Model file for the job. Use its own axes, mm. A direction names the side the tool comes from. Round coordinates to 2 decimals unless told otherwise and drop trailing zeros. Write each loop counter-clockwise with the first axis right and the second up, starting at its lowest first coordinate (ties: lowest second). Pieces come first, ordered by that corner, then holes. Notation, with made-up numbers: (36, 11.5) - (59, 11.5) arc R24 ccw to (59, 36.5) - close; hole circle Ø2 at (52, -9.75). An arc over 180 degrees is marked (long way). One line per item, written item: value.
from build123d import *

# Parameters (mm, degrees)
SKETCH_1_W          = 54
SKETCH_1_H          = 48
EXTRUDE_1_DEPTH     = 1
SKETCH_2_R          = 1.5
CUT_EXTRUDE_1_DEPTH = 37.138621999
FILLET_1_R          = 5
SKETCH_3_W          = 10
SKETCH_3_H          = 7
EXTRUDE_2_DEPTH     = 5
SKETCH_4_W          = 8
SKETCH_4_H          = 8
SKETCH_4_W_2        = 4
SKETCH_4_H_2        = 6
SKETCH_4_H_3        = 4
EXTRUDE_3_DEPTH     = 1


with BuildPart() as part:
    # ｽｹｯﾁ1 → ﾎﾞｽ - 押し出し1 (new body)
    with BuildSketch(Plane.XY):
        Rectangle(SKETCH_1_W, SKETCH_1_H)
    extrude(amount=EXTRUDE_1_DEPTH)

    # ｽｹｯﾁ2 → ｶｯﾄ - 押し出し1 (cut, through all)
    with BuildSketch(Plane.XY.offset(1)):
        with Locations((-24.5, 21)):
            Circle(SKETCH_2_R)
        with Locations((24.5, -21)):
            Circle(SKETCH_2_R)
    extrude(amount=-CUT_EXTRUDE_1_DEPTH, mode=Mode.SUBTRACT)

    # ﾌｨﾚｯﾄ1
    fillet_1_edges = [part.edges().sort_by_distance(p)[0] for p in [
        (27, -24, 0.5),
        (-27, -24, 0.5),
        (-27, 24, 0.5),
        (27, 24, 0.5),
    ]]
    fillet(fillet_1_edges, radius=FILLET_1_R)

    # ｽｹｯﾁ3 → ﾎﾞｽ - 押し出し2 (add)
    with BuildSketch(Plane.XY.offset(1)):
        with Locations((-14, 19.5)):
            Rectangle(SKETCH_3_W, SKETCH_3_H)
        with Locations((0, 19.5)):
            Rectangle(SKETCH_3_W, SKETCH_3_H)
        with Locations((14, 19.5)):
            Rectangle(SKETCH_3_W, SKETCH_3_H)
        with Locations((-14, -19.5)):
            Rectangle(SKETCH_3_W, SKETCH_3_H)
        with Locations((0, -19.5)):
            Rectangle(SKETCH_3_W, SKETCH_3_H)
        with Locations((14, -19.5)):
            Rectangle(SKETCH_3_W, SKETCH_3_H)
    extrude(amount=EXTRUDE_2_DEPTH)

    # ｽｹｯﾁ4 → ﾎﾞｽ - 押し出し3 (add)
    with BuildSketch(Plane.XY.offset(1)):
        with Locations((-10, -8)):
            Rectangle(SKETCH_4_W, SKETCH_4_H)
        with Locations((3, -12)):
            Rectangle(SKETCH_4_W_2, SKETCH_4_H_2)
        with Locations((6, 8)):
            Rectangle(SKETCH_4_W_2, SKETCH_4_H_3)
    extrude(amount=EXTRUDE_3_DEPTH)


solid = part.part
1. Band-saw the part on C-C on y = 21. Write the cut outline in (x, z), plus the area to 3 significant figures.
Report:
outline: (-26.58, 0) - (-26, 0) - (-26, 1) - (-26.58, 1) - close; (-23, 0) - (26.58, 0) - (26.58, 1) - (19, 1) - (19, 6) - (9, 6) - (9, 1) - (5, 1) - (5, 6) - (-5, 6) - (-5, 1) - (-9, 1) - (-9, 6) - (-19, 6) - (-19, 1) - (-23, 1) - close
area: 200 mm²
2. Band-saw the part on D-D on x = 13. Write the cut outline in (y, z).
Report:
outline: (-24, 0) - (24, 0) - (24, 1) - (23, 1) - (23, 6) - (16, 6) - (16, 1) - (-16, 1) - (-16, 6) - (-23, 6) - (-23, 1) - (-24, 1) - close
3. Band-saw the part on A-A on x = -24.5. Write the cut outline in (y, z).
Report:
outline: (-23.33, 0) - (19.5, 0) - (19.5, 1) - (-23.33, 1) - close; (22.5, 0) - (23.33, 0) - (23.33, 1) - (22.5, 1) - close
4. Mould opens along X. For faces 5 (the face through (5, 19, 3)), 6 (the face through (-5, 19, 3)), 7 (the face through (-25.57, -22.5, 0.51)), 8 (the face through (-14, -16, 3)) say: released by +X, released by -X, zero draft, split by the parting line, or undercut.
Report:
face 5: undercut
face 6: undercut
face 7: released by -X
face 8: zero draft
5. Band-saw the part on B-B on y = -8. Write the cut outline in (x, z).
Report:
outline: (-27, 0) - (27, 0) - (27, 1) - (-6, 1) - (-6, 2) - (-14, 2) - (-14, 1) - (-27, 1) - close
6. Drop flat-ended pins along their axis: pin 1 (1.5 mm diameter, centred on y = -20.5, z = 4, fed in from -X); pin 2 (2.5 mm diameter, centred on x = 13, z = 4, fed in from +Y); pin 3 (1.5 mm diameter, centred on x = -12, z = 3.5, fed in from -Y). Give the stop position or say it passes through.
Report:
pin 1: x = -19
pin 2: y = 23
pin 3: y = -23
7. Tool access for faces 1 (the face through (-14, 16, 3)), 2 (the face through (0, -23, 3)), 3 (the face through (-14, 23, 3)), 4 (the face through (-5, -20, 3)): list every direction of +Z, -Z, +X, -X, +Y, -Y with a clear straight run to the whole face (end or side of a thin tool).
Report:
face 1: +Z, +X, -X
face 2: +Z, +X, -X, -Y
face 3: +Z, +X, -X, +Y
face 4: +Z, +Y, -Y
8. Wall check: probe 1 along X at (y, z) = (-20, 3.05); probe 2 along Y at (x, z) = (-11, 3.75); probe 3 along Z at (x, y) = (21.5, -16.5). Give the ranges that are in metal, low to high. Write a range as [from, to].
Report:
probe 1: [-19, -9], [-5, 5], [9, 19]
probe 2: [-23, -16], [16, 23]
probe 3: [0, 1]
